Verification items for this drawing (mm, ordinates from the low corner). A direction names the side the tool comes from. Coordinates: 2 decimals unless noted, no trailing zeros. Order: outer loops, then holes, each group sorted by start corner. A loop starts at its lowest first (then second) coordinate and runs counter-clockwise, first axis right, second up.
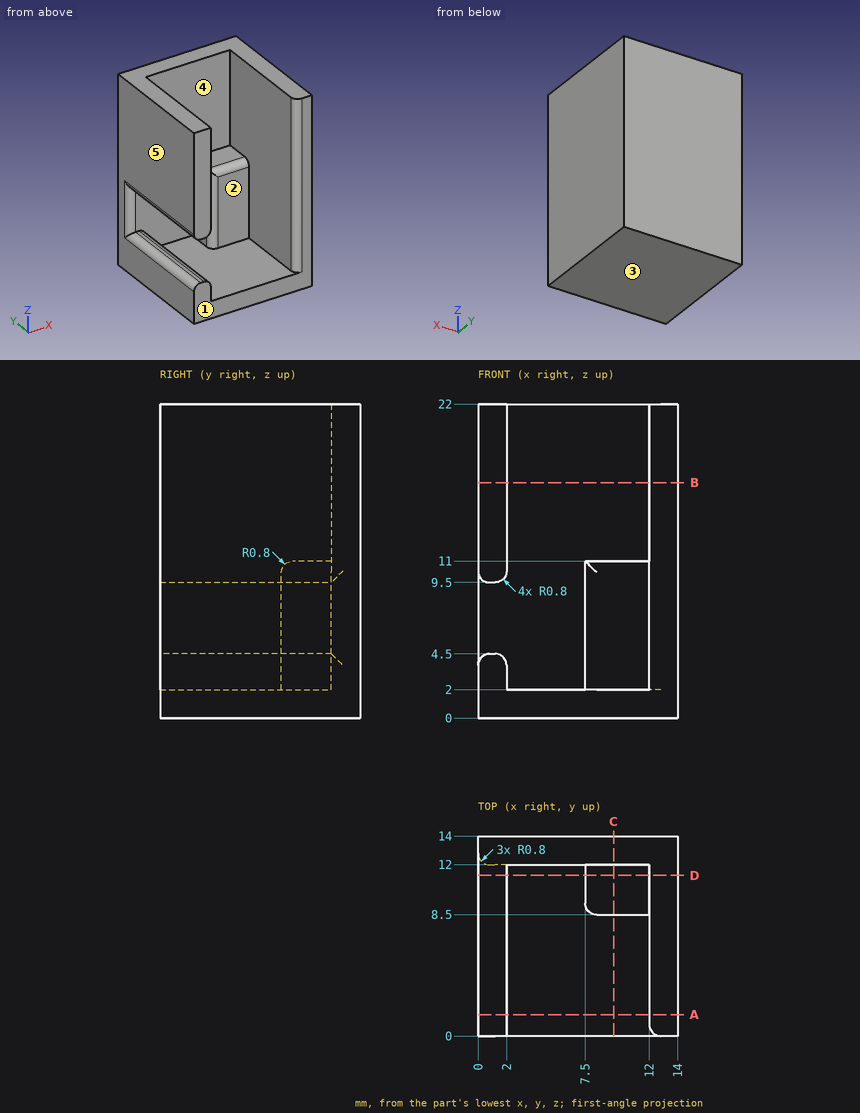
(1) Cross-section at C-C (x = 9.5). Enter the section's corners in (y, z), and give its area (3 significant figures).
Filled in:
outline: (0, 0) - (14, 0) - (14, 22) - (12, 22) - (12, 11) - (9.3, 11) arc R0.8 ccw to (8.5, 10.2) - (8.5, 2) - (0, 2) - close
area: 99.4 mm2
(2) Cross-section at A-A (y = 1.5). Enter the section's corners in (x, z), and give its area (3 significant figures).
Filled in:
outline: (0, 0) - (14, 0) - (14, 22) - (12, 22) - (12, 2) - (2, 2) - (2, 3.7) arc R0.8 ccw to (1.2, 4.5) - (0.8, 4.5) arc R0.8 ccw to (0, 3.7) - close; (0, 10.3) arc R0.8 ccw to (0.8, 9.5) - (1.2, 9.5) arc R0.8 ccw to (2, 10.3) - (2, 22) - (0, 22) - close
area: 97.5 mm2
(3) Cross-section at B-B (z = 16.5). Enter the section's corners in (x, y), and give its area (3 significant figures).
Filled in:
outline: (0, 0) - (2, 0) - (2, 12) - (12, 12) - (12, 0.8) arc R0.8 ccw to (12.8, 0) - (14, 0) - (14, 14) - (0, 14) - close
area: 75.9 mm2
(4) Release check for a two-part mould opening along X. For the marked faces 3, 4 and 5 record: +X half, -X half, draft (parallel to the pull), parting line (faces both ways), or undercut.
Filled in:
face 3: draft
face 4: undercut
face 5: -X half
(5) Thickness scan on probe 1 along X at (y, z) = (1.5, 17.75); probe 2 along Z at (x, y) = (1, 8); probe 3 along Y at (x, z) = (10.5, 19.75). Record the ranges inside material, lowest first.
Filled in:
probe 1: x = 0 to 2, 12 to 14
probe 2: z = 0 to 4.5, 9.5 to 22
probe 3: y = 12 to 14
(6) Go/stop test with flat-tipped pins: P1, Ø1, axis at x = 8.5, z = 3, coming from the -Y side; P2, Ø0.8, axis at x = 10.5, y = 10, coming from the +Z side; P3, Ø2, axis at y = 11, z = 5, coming from the -X side. Record where each tip stops, or that it passes through.
Filled in:
P1: stops at y = 8.5
P2: stops at z = 11
P3: stops at x = 0.06
(7) Tool access check on the marked faces 1 and 2. Record the directions out of +Z, -Z, +X, -X, +Y, -Y that give a thin tool (end or side, any length) a straight path to the whole face; none if there is none.
Filled in:
face 1: +Z, -Z, +X, -X, -Y
face 2: +Z, -Y
(8) Cross-section at D-D (y = 11.25). Enter the section's corners in (x, z).
Filled in:
outline: (0, 0) - (14, 0) - (14, 22) - (12, 22) - (12, 11) - (7.5, 11) - (7.5, 2) - (2, 2) - (2, 3.7) arc R0.8 ccw to (1.2, 4.5) - (0.8, 4.5) arc R0.8 ccw to (0, 3.7) - close; (0, 10.3) arc R0.8 ccw to (0.8, 9.5) - (1.2, 9.5) arc R0.8 ccw to (2, 10.3) - (2, 22) - (0, 22) - close
